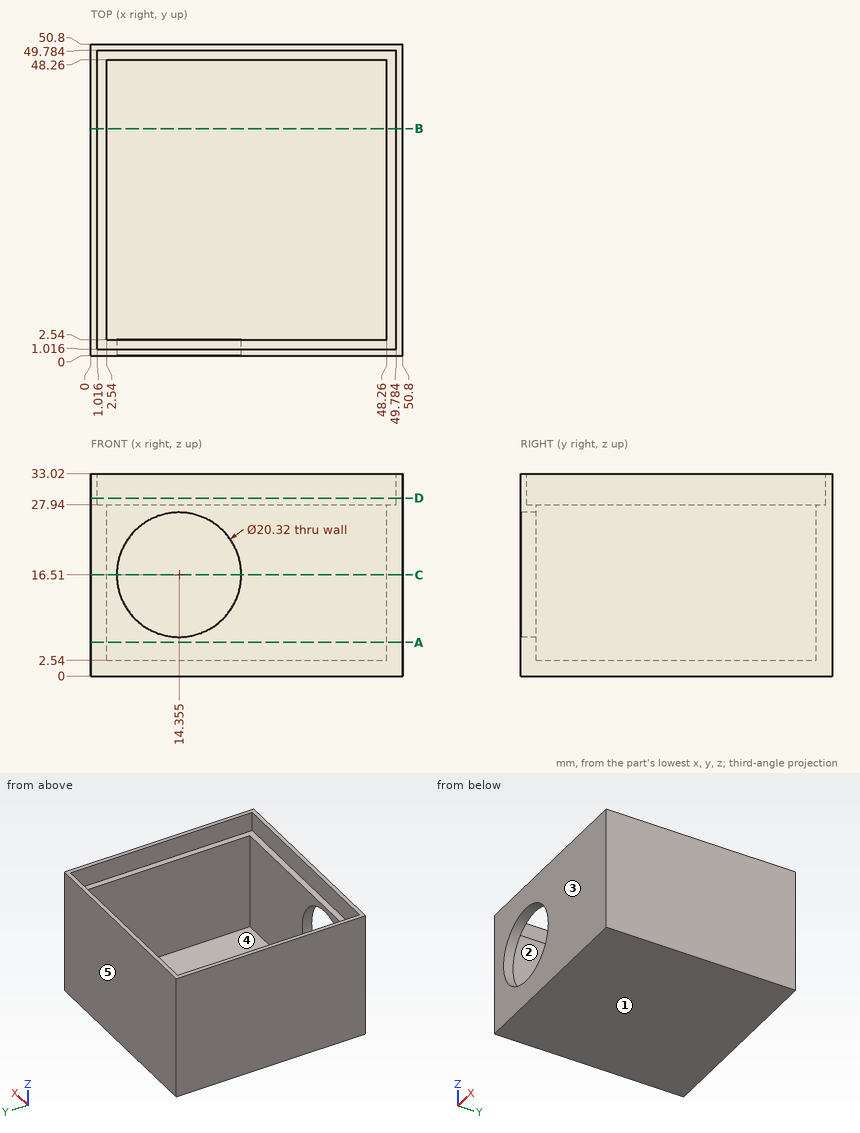
Design review of the part shown in the three views and the two pictorial views. Dimensions are in mm from the part's minimum x, y and z. A direction names the side the tool comes from. Round coordinates to 2 decimals unless told otherwise and drop trailing zeros. Loops run counter-clockwise (first coordinate to the right, second up) from the corner with the lowest first, then second, coordinate; pieces in that order, holes last.
(1) Mouldability with a two-part tool opening along Y and no side actions: class the marked faces 1, 2 and 3 as released by +Y, released by -Y, zero draft, split by the parting line, or undercut.
Returned:
face 1: zero draft
face 2: undercut
face 3: released by -Y
(2) We need section B-B (y = 37). Give the boundary of the cut face in (x, z).
Returned:
outline: (0, 0) - (50.8, 0) - (50.8, 33.02) - (49.78, 33.02) - (49.78, 27.94) - (48.26, 27.94) - (48.26, 2.54) - (2.54, 2.54) - (2.54, 27.94) - (1.02, 27.94) - (1.02, 33.02) - (0, 33.02) - close
(3) We need section A-A (z = 5.5). Give the boundary of the cut face in (x, y).
Returned:
outline: (0, 0) - (50.8, 0) - (50.8, 50.8) - (0, 50.8) - close; hole (2.54, 2.54) - (48.26, 2.54) - (48.26, 48.26) - (2.54, 48.26) - close
(4) Tool access review of the marked faces 4 and 5: name each direction out of +Z, -Z, +X, -X, +Y, -Y from which nothing blocks a thin tool from reaching the whole face with its end or side.
Returned:
face 4: +Z
face 5: +Z, -Z, +X, -X, +Y
(5) We need section D-D (z = 29). Give the boundary of the cut face in (x, y), plus the area to 3 significant figures.
Returned:
outline: (0, 0) - (50.8, 0) - (50.8, 50.8) - (0, 50.8) - close; hole (1.02, 1.02) - (49.78, 1.02) - (49.78, 49.78) - (1.02, 49.78) - close
area: 202 mm2
(6) We need section C-C (z = 16.51). Give the boundary of the cut face in (x, y) (3 decimals).
Returned:
outline: (0, 0) - (4.195, 0) - (4.195, 2.54) - (2.54, 2.54) - (2.54, 48.26) - (48.26, 48.26) - (48.26, 2.54) - (24.515, 2.54) - (24.515, 0) - (50.8, 0) - (50.8, 50.8) - (0, 50.8) - close
(7) Wall thickness on line 1 along Y through (x, z) = (7, 5.5); line 2 along X through (y, z) = (30.5, 30.5): over which ranges is each line inside the solid? List them lowest first.
Returned:
line 1: y = 0 to 2.54, 48.26 to 50.8
line 2: x = 0 to 1.02, 49.78 to 50.8
(8) Clearance check with flat-ended pins moving along their axes: P1, Ø4, axis at y = 13.5, z = 29, coming from the -X side; P2, Ø13.5, axis at x = 19.5, y = 33, coming from the +Z side. State where each tip first meets the part, or that it passes through.
Returned:
P1: stops at x = 0
P2: stops at z = 2.54
